Verification items for this drawing (mm, ordinates from the low corner). A direction names the side the tool comes from. Round coordinates to 2 decimals unless told otherwise and drop trailing zeros. Order: outer loops, then holes, each group sorted by start corner. A loop starts at its lowest first (then second) coordinate and runs counter-clockwise, first axis right, second up. Notation, with made-up numbers: (75, 32.25) -> (82, 32.25) arc R23 cw to (82, 58.25) -> close; hole circle Ø5 at (87, 48). An arc over 180 degrees is marked (long way). Put each result on its own line as item: value.
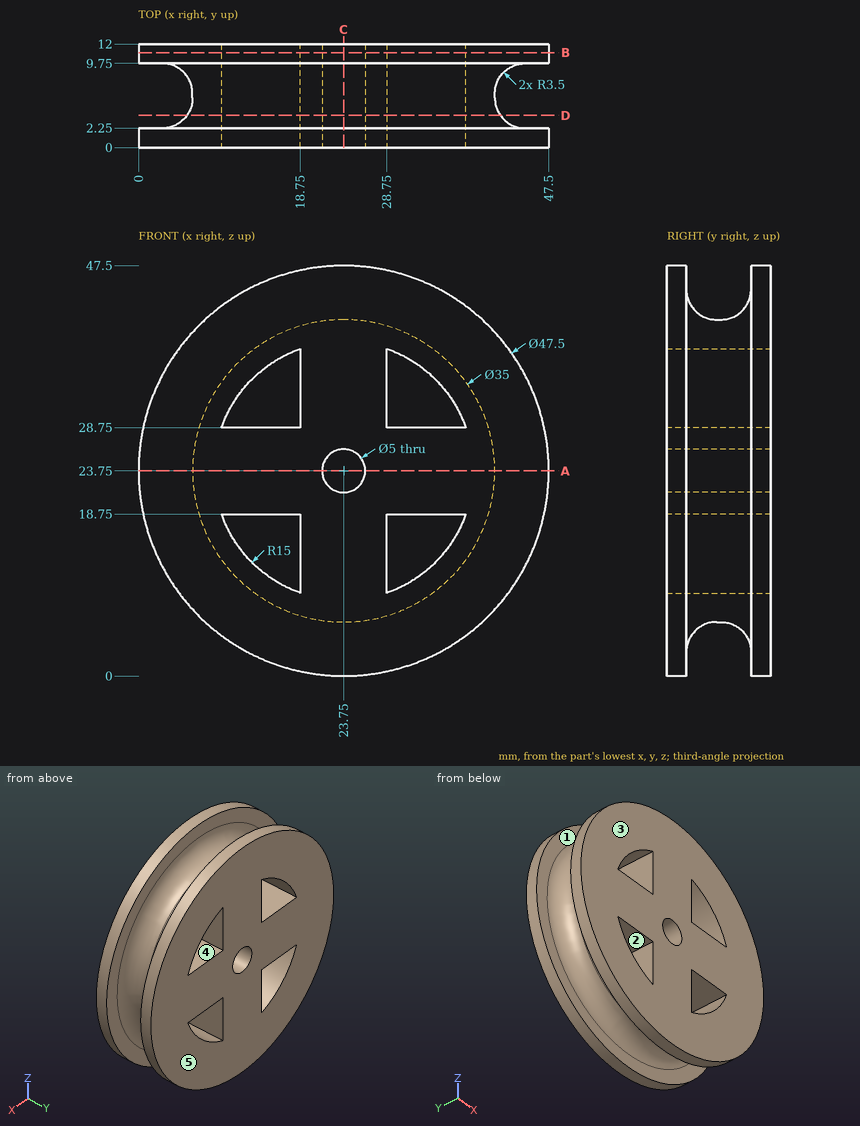
Item 1: Tool access check on the marked faces 4 and 5. Record the directions out of +Z, -Z, +X, -X, +Y, -Y that give a thin tool (end or side, any length) a straight path to the whole face; none if there is none.
Check sheet entries:
face 4: +Y, -Y
face 5: +Z, -Z, +X, -X, +Y
Item 2: Section check D-D on y = 3.75. Record the boundary of the cut face in (x, z).
Check sheet entries:
outline: circle Ø36.26 at (23.75, 23.75); hole (9.61, 18.75) arc R15 ccw to (18.75, 9.61) -> (18.75, 18.75) -> close; hole (9.61, 28.75) -> (18.75, 28.75) -> (18.75, 37.89) arc R15 ccw to start; hole circle Ø5 at (23.75, 23.75); hole (28.75, 9.61) arc R15 ccw to (37.89, 18.75) -> (28.75, 18.75) -> close; hole (28.75, 28.75) -> (37.89, 28.75) arc R15 ccw to (28.75, 37.89) -> close
Item 3: Material ranges on L1, parallel to Z at x = 30, y = 1.5; L2, parallel to Z at x = 23.75, y = 5.5; L3, parallel to X at y = 4.75, z = 36, recorded low to high. Write a range as [from, to].
Check sheet entries:
L1: z = [0.84, 10.11], [18.75, 28.75], [37.39, 46.66]
L2: z = [6.24, 21.25], [26.25, 41.26]
L3: x = [11.05, 15.09], [18.75, 28.75], [32.41, 36.45]
Item 4: Release check for a two-part mould opening along Y. For the marked faces 1, 2 and 3 record: +Y half, -Y half, draft (parallel to the pull), parting line (faces both ways), or undercut.
Check sheet entries:
face 1: undercut
face 2: draft
face 3: -Y half
Item 5: Gauge pin test, flat ends, axial feed: pin 1 Ø2.5 at (y, z) = (9, 32) entering from -X; pin 2 Ø4.5 at (x, y) = (14.5, 8.5) entering from +Z; pin 3 Ø1 at (y, z) = (8.5, 17) entering from -X. Record the tip position at first contact, or that the pin passes through.
Check sheet entries:
pin 1: stops at x = 1.13
pin 2: stops at z = 46.32
pin 3: stops at x = 6.14
Item 6: Section check C-C on x = 23.75. Record the boundary of the cut face in (y, z).
Check sheet entries:
outline: (0, 0) -> (2.25, 0) -> (2.25, 2.75) arc R3.5 cw to (5.75, 6.25) -> (6.25, 6.25) arc R3.5 cw to (9.75, 2.75) -> (9.75, 0) -> (12, 0) -> (12, 21.25) -> (0, 21.25) -> close; (0, 26.25) -> (12, 26.25) -> (12, 47.5) -> (9.75, 47.5) -> (9.75, 44.75) arc R3.5 cw to (6.25, 41.25) -> (5.75, 41.25) arc R3.5 cw to (2.25, 44.75) -> (2.25, 47.5) -> (0, 47.5) -> close
Item 7: Section check B-B on y = 11. Record the boundary of the cut face in (x, z).
Check sheet entries:
outline: circle Ø47.5 at (23.75, 23.75); hole (9.61, 18.75) arc R15 ccw to (18.75, 9.61) -> (18.75, 18.75) -> close; hole (9.61, 28.75) -> (18.75, 28.75) -> (18.75, 37.89) arc R15 ccw to start; hole circle Ø5 at (23.75, 23.75); hole (28.75, 9.61) arc R15 ccw to (37.89, 18.75) -> (28.75, 18.75) -> close; hole (28.75, 28.75) -> (37.89, 28.75) arc R15 ccw to (28.75, 37.89) -> close
Item 8: Section check A-A on z = 23.75. Record the boundary of the cut face in (x, y), then the cut area to 3 significant figures.
Check sheet entries:
outline: (0, 0) -> (21.25, 0) -> (21.25, 12) -> (0, 12) -> (0, 9.75) -> (2.75, 9.75) arc R3.5 cw to (6.25, 6.25) -> (6.25, 5.75) arc R3.5 cw to (2.75, 2.25) -> (0, 2.25) -> close; (26.25, 0) -> (47.5, 0) -> (47.5, 2.25) -> (44.75, 2.25) arc R3.5 cw to (41.25, 5.75) -> (41.25, 6.25) arc R3.5 cw to (44.75, 9.75) -> (47.5, 9.75) -> (47.5, 12) -> (26.25, 12) -> close
area: 427 mm^2
